from build123d import *

# Parameters (mm, degrees)
SKETCH1_R             = 14.29385
SKETCH1_R_2           = 11.1125
BOSS_EXTRUDE1_DEPTH   = 6.35
CROQUIS1_R            = 2.38125
CORTAR_EXTRUIR1_DEPTH = 50
CROQUIS2_R            = 5
CORTAR_EXTRUIR2_DEPTH = 3.175


with BuildPart() as part:
    # Sketch1 → Boss-Extrude1 (new body)
    with BuildSketch(Plane.XY):
        with BuildLine():
            Line((0, 70), (310, 45))
            ThreePointArc((310, 45), (355, 0), (310, -45))
            Line((310, -45), (5.171398252, -69.808714643))
            ThreePointArc((5.171398252, -69.808714643), (-69.952162315, -2.587467389), (0, 70))
        make_face()
        Circle(SKETCH1_R, mode=Mode.SUBTRACT)
        with Locations((310, 0)):
            Circle(SKETCH1_R, mode=Mode.SUBTRACT)
        with Locations((162.878542763, 35)):
            Circle(SKETCH1_R_2, mode=Mode.SUBTRACT)
        with BuildLine():
            Line((107.898974887, 49.259511156), (143.314248041, 46.40344074))
            ThreePointArc((143.314248041, 46.40344074), (147.389908855, 43.644764005), (147.127454118, 38.730252238))
            Line((147.127454118, 38.730252238), (129.916226305, 11.754586611))
            ThreePointArc((129.916226305, 11.754586611), (125.651076231, 9.444205574), (121.433006579, 11.839462159))
            Line((121.433006579, 11.839462159), (103.228961238, 41.671198203))
            ThreePointArc((103.228961238, 41.671198203), (103.238833139, 46.896293531), (107.898974887, 49.259511156))
        make_face(mode=Mode.SUBTRACT)
        with BuildLine():
            Line((70.523244027, 6), (102.03004784, 6))
            ThreePointArc((102.03004784, 6), (106.3902351, 8.552804247), (106.298140539, 13.604493178))
            Line((106.298140539, 13.604493178), (88.746497295, 42.367110417))
            ThreePointArc((88.746497295, 42.367110417), (67.562092561, 48.186702797), (60.457600585, 27.397935321))
            ThreePointArc((60.457600585, 27.397935321), (63.602250375, 18.987418874), (65.58297828, 10.229432452))
            ThreePointArc((65.58297828, 10.229432452), (67.271539685, 7.201787411), (70.523244027, 6))
        make_face(mode=Mode.SUBTRACT)
        with BuildLine():
            Line((219.623774494, 32.810522613), (206.130928429, 12.417497436))
            ThreePointArc((206.130928429, 12.417497436), (201.919524559, 10.176643248), (197.745901529, 12.48710226))
            Line((197.745901529, 12.48710226), (183.296864227, 35.133505128))
            ThreePointArc((183.296864227, 35.133505128), (183.227765467, 40.400743015), (187.913912204, 42.80669363))
            Line((187.913912204, 42.80669363), (215.855795571, 40.553315939))
            ThreePointArc((215.855795571, 40.553315939), (219.949772588, 37.757395035), (219.623774494, 32.810522613))
        make_face(mode=Mode.SUBTRACT)
        with BuildLine():
            Line((88.746497295, -42.367110417), (106.298140539, -13.604493178))
            ThreePointArc((106.298140539, -13.604493178), (106.3902351, -8.552804247), (102.03004784, -6))
            Line((102.03004784, -6), (70.523244027, -6))
            ThreePointArc((70.523244027, -6), (67.271539685, -7.201787411), (65.58297828, -10.229432452))
            ThreePointArc((65.58297828, -10.229432452), (63.602250375, -18.987418874), (60.457600585, -27.397935321))
            ThreePointArc((60.457600585, -27.397935321), (67.562092561, -48.186702797), (88.746497295, -42.367110417))
        make_face(mode=Mode.SUBTRACT)
        with BuildLine():
            Line((187.913912204, -42.80669363), (215.855795571, -40.553315939))
            ThreePointArc((215.855795571, -40.553315939), (219.949772588, -37.757395035), (219.623774494, -32.810522613))
            Line((219.623774494, -32.810522613), (206.130928429, -12.417497436))
            ThreePointArc((206.130928429, -12.417497436), (201.919524559, -10.176643248), (197.745901529, -12.48710226))
            Line((197.745901529, -12.48710226), (183.296864227, -35.133505128))
            ThreePointArc((183.296864227, -35.133505128), (183.227765467, -40.400743015), (187.913912204, -42.80669363))
        make_face(mode=Mode.SUBTRACT)
        with BuildLine():
            Line((121.433006579, -11.839462159), (103.228961238, -41.671198203))
            ThreePointArc((103.228961238, -41.671198203), (103.238833139, -46.896293531), (107.898974887, -49.259511156))
            Line((107.898974887, -49.259511156), (143.314248041, -46.40344074))
            ThreePointArc((143.314248041, -46.40344074), (147.389908855, -43.644764005), (147.127454118, -38.730252238))
            Line((147.127454118, -38.730252238), (129.916226305, -11.754586611))
            ThreePointArc((129.916226305, -11.754586611), (125.651076231, -9.444205574), (121.433006579, -11.839462159))
        make_face(mode=Mode.SUBTRACT)
    extrude(amount=BOSS_EXTRUDE1_DEPTH)

    # Croquis1 → Cortar-Extruir1 (cut)
    with BuildSketch(Plane.XY.offset(6.35)):
        with Locations((98.995555235, -37.090103176)):
            Circle(CROQUIS1_R)
        with Locations((228.877351461, -26.519571404)):
            Circle(CROQUIS1_R)
    extrude(amount=-CORTAR_EXTRUIR1_DEPTH, mode=Mode.SUBTRACT)

    # Croquis2 → Cortar-Extruir2 (cut)
    with BuildSketch(Plane.XY.offset(6.35)):
        with Locations((98.995555235, -37.090103176)):
            Circle(CROQUIS2_R)
        with Locations((228.877351461, -26.519571404)):
            Circle(CROQUIS2_R)
    extrude(amount=-CORTAR_EXTRUIR2_DEPTH, mode=Mode.SUBTRACT)


solid = part.part
For this review, take the finished solid that the model builds, in its own axes (mm). A direction names the side the tool comes from. Round coordinates to 2 decimals unless told otherwise and drop trailing zeros. Loops run counter-clockwise (first coordinate to the right, second up) from the corner with the lowest first, then second, coordinate; pieces in that order, holes last. Notation, with made-up numbers: (21, 39) - (35, 39) arc R20 ccw to (35, 57) - close; hole circle Ø8 at (29.25, -22). An arc over 180 degrees is marked (long way). One line per item, written item: value. Start each with the question number.
Item 1: Take a section at B-B (x = -5.5). Give the boundary of the cut face in (y, z), plus the area to 3 significant figures.
Item 2: Take a section at C-C (z = 4.5). State how many separate pieces and enclosed holes the cut face has, plus the area to 3 significant figures.
Item 3: For L1, parallel to X at y = 1, z = 5; L2, parallel to Y at x = 184.5, z = 4; L3, parallel to X at y = -2.5, z = 0.5, list the stretches that pass through material, from the lowest coordinate up.
Item 4: Take a section at A-A (y = 0). Give the boundary of the cut face in (x, z).
Item 5: The part is to be moulded in two halves that separate along Y. For faces 3 (the cylindrical face through (354.99, 0.99, 3.13)), 4 (the cylindrical face through (-1.861, 14.172, 3.131)), 5 (the cylindrical face through (67.264, -48.025, 3.131)), 6 (the flat face through (152.83, 57.675, 3.131)), say which applies: +Y half, -Y half, draft (parallel to the pull), parting line (faces both ways), or undercut.
Item 6: For faces 1 (the flat face through (230, -29, 3.175)), 2 (the flat face through (97.65, 27.78, 3.13)), list the 3-axis set-ups (+Z, -Z, +X, -X, +Y, -Y) from which the entire face can be reached by the end or side of a thin tool; tool diameter is ignored.
Item 7: Clearance check with flat-ended pins moving along their axes: pin 1 Ø9 at (x, y) = (228.88, -26.52) entering from +Z (3 decimals); pin 2 Ø10 at (x, y) = (103, 17) entering from +Z; pin 3 Ø1.9 at (x, z) = (93, 4.5) entering from -Y; pin 4 Ø1.9 at (x, z) = (83.5, 2) entering from +Y. State where each tip first meets the part, or that it passes through.
Item 8: Take a section at D-D (x = 264.5). Give the boundary of the cut face in (y, z).
Answer below:
1. outline: (-69.78, 0) - (-13.19, 0) - (-13.19, 6.35) - (-69.78, 6.35) - close; (13.19, 0) - (69.78, 0) - (69.78, 6.35) - (13.19, 6.35) - close
1. area: 719 mm2
2. separate pieces: 1
2. enclosed holes: 11
2. area: 38,000 mm2
3. L1: x = -69.99 to -14.26, 14.26 to 295.74, 324.26 to 354.99
3. L2: y = -55.21 to -41.81, -33.25 to 33.25, 41.81 to 55.12
3. L3: x = -69.96 to -14.07, 14.07 to 295.93, 324.07 to 354.93
4. outline: (-70, 0) - (-14.29, 0) - (-14.29, 6.35) - (-70, 6.35) - close; (14.29, 0) - (295.71, 0) - (295.71, 6.35) - (14.29, 6.35) - close; (324.29, 0) - (355, 0) - (355, 6.35) - (324.29, 6.35) - close
5. face 3: parting line
5. face 4: undercut
5. face 5: undercut
5. face 6: +Y half
6. face 1: +Z
6. face 2: +Z, -Z
7. pin 1: stops at z = 3.175
7. pin 2: stops at z = 6.35
7. pin 3: stops at y = -62.74
7. pin 4: stops at y = 63.34
8. outline: (-48.7, 0) - (48.67, 0) - (48.67, 6.35) - (-48.7, 6.35) - close
